from build123d import *

# Parameters (mm, degrees)
REVOLUCI_N1_ANGLE         = 180
CROQUIS2_W                = 8
CROQUIS2_H                = 33.6
SALIENTE_EXTRUIR1_DEPTH   = 14
SALIENTE_EXTRUIR1_2_DEPTH = 14
SALIENTE_EXTRUIR2_START   = -33.6
SALIENTE_EXTRUIR2_DEPTH   = 33.6
CROQUIS4_R                = 2
CORTAR_EXTRUIR1_DEPTH     = 26


# Read off the part's stored shape, not the designer's step: Saliente-Extruir2
with BuildPart() as part:
    # Croquis1 → Revolución1 (revolve)
    with BuildSketch(Plane.XY):
        Polygon((-8, 0), (-5, 0), (-5, 3), (-14, 3), (-14, -30.6), (-5, -30.6), (-5, -26.6), (-8, -26.6), align=None)
    revolve(axis=Axis((0, 0, 0), (0, -1, 0)), revolution_arc=REVOLUCI_N1_ANGLE)



with BuildPart() as body_2:
    # Croquis2 → Saliente-Extruir1 (new body)
    with BuildSketch(Plane.XY):
        with Locations((-12, -13.8)):
            Rectangle(CROQUIS2_W, CROQUIS2_H)
    extrude(amount=-SALIENTE_EXTRUIR1_DEPTH)


with BuildPart() as body_3:
    # Croquis2 → Saliente-Extruir1 2 (new body)
    with BuildSketch(Plane.XY):
        with Locations((12, -13.8)):
            Rectangle(CROQUIS2_W, CROQUIS2_H)
    extrude(amount=-SALIENTE_EXTRUIR1_2_DEPTH)


with BuildPart() as part_1:
    add(part.part)

    add(body_2.part)  # Saliente-Extruir2 merges body 2

    add(body_3.part)  # Saliente-Extruir2 merges body 3
    # Saliente-Extruir2 outline → Saliente-Extruir2 (add)
    with BuildSketch(Plane(origin=(0, 3, 0), x_dir=(1, 0, 0), z_dir=(0, 1, 0)).offset(SALIENTE_EXTRUIR2_START)):
        with BuildLine():
            Line((8, 14), (0, 14))
            ThreePointArc((0, 14), (4.192388692, 13.357540082), (8, 11.489125293))
            Line((8, 11.489125293), (8, 14))
        make_face()
        with BuildLine():
            Line((0, 14), (-8, 14))
            Line((-8, 14), (-8, 11.489125293))
            ThreePointArc((-8, 11.489125293), (-4.192388692, 13.357540082), (0, 14))
        make_face()
    extrude(amount=SALIENTE_EXTRUIR2_DEPTH)

    # Croquis4 → Cortar-Extruir1 (cut)
    with BuildSketch(Plane.XY):
        with Locations((-12, -2)):
            Circle(CROQUIS4_R)
        with Locations((12, -2)):
            Circle(CROQUIS4_R)
        with Locations((-12, -25.6)):
            Circle(CROQUIS4_R)
        with Locations((12, -25.6)):
            Circle(CROQUIS4_R)
    extrude(amount=-CORTAR_EXTRUIR1_DEPTH, mode=Mode.SUBTRACT)


solid = part_1.part
Geometry check sheet. Reference: the model listing, model coordinates, mm. A direction names the side the tool comes from. Coordinates: 2 decimals unless noted, no trailing zeros. Order: outer loops, then holes, each group sorted by start corner. A loop starts at its lowest first (then second) coordinate and runs counter-clockwise, first axis right, second up. Notation, with made-up numbers: (-16, 32) - (22, 32) arc R36 cw to (22, 67) - close; hole circle Ø8 at (9.5, -5). An arc over 180 degrees is marked (long way). One line per item, written item: value.
(1) Release check for a two-part mould opening along Y. For faces 1 (the face through (0, 2, -5)), 2 (the face through (-13.6, -3.2, -6.9)), 3 (the face through (0, -30.6, -7)) record: +Y half, -Y half, draft (parallel to the pull), parting line (faces both ways), or undercut.
Data:
face 1: draft
face 2: undercut
face 3: -Y half
(2) Sectioned sample at D-D (z = -10). Enter the section's corners in (x, y).
Data:
outline: (-16, -30.6) - (16, -30.6) - (16, 3) - (-16, 3) - close; hole circle Ø4 at (-12, -25.6); hole circle Ø4 at (-12, -2); hole circle Ø4 at (12, -25.6); hole circle Ø4 at (12, -2)
(3) Access from +Z, -Z, +X, -X, +Y, -Y to the whole of each face (thin tool, end or side, straight path). Record for faces 4 (the face through (0, -14, -14)), 5 (the face through (0, -26.6, -6)).
Data:
face 4: -Z, +X, -X, +Y, -Y
face 5: +Z
(4) Depth check by flat-ended pin: pin 1 Ø3.5 at (x, y) = (-12, -2) entering from -Z. Enter the tip coordinate at first touch or a pass-through.
Data:
pin 1: passes through
(5) Sectioned sample at C-C (z = -4). Enter the section's corners in (x, y).
Data:
outline: (-16, -30.6) - (-3, -30.6) - (-3, -26.6) - (-6.93, -26.6) - (-6.93, 0) - (-3, 0) - (-3, 3) - (-16, 3) - close; (3, -30.6) - (16, -30.6) - (16, 3) - (3, 3) - (3, 0) - (6.93, 0) - (6.93, -26.6) - (3, -26.6) - close; hole circle Ø4 at (-12, -25.6); hole circle Ø4 at (-12, -2); hole circle Ø4 at (12, -25.6); hole circle Ø4 at (12, -2)
(6) Sectioned sample at B-B (x = 12). Enter the section's corners in (y, z).
Data:
outline: (-30.6, -14) - (-27.6, -14) - (-27.6, 0) - (-30.6, 0) - close; (-23.6, -14) - (-4, -14) - (-4, 0) - (-23.6, 0) - close; (0, -14) - (3, -14) - (3, 0) - (0, 0) - close
(7) Thickness scan on probe 1 along Y at (x, z) = (12, -5.75); probe 2 along X at (y, z) = (-3, -11.5); probe 3 along Y at (x, z) = (-1.5, -6.75). Record the ranges inside material, lowest first. Write a range as from..to.
Data:
probe 1: y = -30.6..-27.6, -23.6..-4, 0..3
probe 2: x = -16..-13.73, -10.27..10.27, 13.73..16
probe 3: y = -30.6..-26.6, 0..3
(8) Sectioned sample at A-A (y = -2). Enter the section's corners in (x, z), and give its area (3 significant figures).
Data:
outline: (-16, -14) - (-14, -14) - (-14, 0) - (-16, 0) - close; (-10, -14) - (10, -14) - (10, 0) - (8, 0) arc R8 cw to (-8, 0) - (-10, 0) - close; (14, -14) - (16, -14) - (16, 0) - (14, 0) - close
area: 235 mm^2
